Verification items for the finished model (mm, model axes). A direction names the side the tool comes from. Coordinates: 2 decimals unless noted, no trailing zeros. Order: outer loops, then holes, each group sorted by start corner. A loop starts at its lowest first (then second) coordinate and runs counter-clockwise, first axis right, second up. Notation, with made-up numbers: (74, 51) -> (118, 51) arc R33 cw to (118, 88) -> close; hole circle Ø5 at (-12, 54). An arc over 180 degrees is marked (long way). Write item = value, one per line. Start each with the question number.
1. Cross-section at C-C on z = 4.5. Record the cut outline in (x, y), plus the area to 3 significant figures.
2. Cross-section at D-D on x = -6. Record the cut outline in (y, z).
3. Release check for a two-part mould opening along Y. For faces 3 (the cylindrical face through (-19.98, -0.88, 3.54)), 4 (the cylindrical face through (-0.715, -7.375, 3.451)), 5 (the flat face through (-5, 5, 0)) record: +Y half, -Y half, draft (parallel to the pull), parting line (faces both ways), or undercut.
4. Thickness scan on line 1 along Z through (x, y) = (-2.5, 21.5); line 2 along Y through (x, z) = (-5, 2); line 3 along Y through (x, z) = (-6, 1.5). Record the ranges inside material, lowest first. Write a range as from..to.
5. Cross-section at A-A on y = 0. Record the cut outline in (x, z), plus the area to 3 significant figures.
6. Set-up check for faces 1 (the flat face through (-11, -17, 1)), 2 (the cylindrical face through (23.846, -7.509, 6.507)): record each of +Z, -Z, +X, -X, +Y, -Y from which the full face is reachable in a straight line by a thin tool's end or side.
7. Go/stop test with flat-tipped pins: P1, Ø1, axis at x = -1.5, z = 2.5, coming from the +Y side (3 decimals); P2, Ø4, axis at y = 7, z = 3.5, coming from the +X side; P3, Ø1.9, axis at x = 0, y = -6, coming from the +Z side; P4, Ø4, axis at x = -16.5, z = 1.5, coming from the -Y side. Record where each tip stops, or that it passes through.
from build123d import *

# Parameters (mm, degrees)
SKETCH4_R          = 1.55
SKETCH4_R_2        = 2.45
CUT_EXTRUDE1_DEPTH = 37.041642582


with BuildPart() as part:
    # Sketch3 → Revolve2 (revolve)
    with BuildSketch(Plane(origin=(0, 0, 0), x_dir=(1, 0, 0), z_dir=(0, 1, 0)), mode=Mode.PRIVATE) as revolve2_sk:
        Polygon((0, 0), (-25, 0), (-25, -1), (-20, -1), (-20, -6), (-25, -6), (-25, -7), (0, -7), align=None)
    revolve(revolve2_sk.sketch.rotate(Axis((0, 0, 7), (0, 0, -1)), 180), axis=Axis((0, 0, 7), (0, 0, -1)))

    # Sketch4 → Cut-Extrude1 (cut, through all)
    with BuildSketch(Plane(origin=(0, 0, 0), x_dir=(-1, 0, 0), z_dir=(0, 0, -1))):
        with Locations((0, 6)):
            Circle(SKETCH4_R)
        with Locations((6, 0)):
            Circle(SKETCH4_R)
        with Locations((0, -6)):
            Circle(SKETCH4_R)
        with Locations((-6, 0)):
            Circle(SKETCH4_R)
        Circle(SKETCH4_R_2)
    extrude(amount=-CUT_EXTRUDE1_DEPTH, mode=Mode.SUBTRACT)


solid = part.part
Worked out:
q1.outline = circle Ø40 at (0, 0); hole circle Ø3.1 at (-6, 0); hole circle Ø4.9 at (0, 0); hole circle Ø3.1 at (0, -6); hole circle Ø3.1 at (0, 6); hole circle Ø3.1 at (6, 0)
q1.area = 1,210 mm²
q2.outline = (-24.27, 0) -> (-1.55, 0) -> (-1.55, 7) -> (-24.27, 7) -> (-24.27, 6) -> (-19.08, 6) -> (-19.08, 1) -> (-24.27, 1) -> close; (1.55, 0) -> (24.27, 0) -> (24.27, 1) -> (19.08, 1) -> (19.08, 6) -> (24.27, 6) -> (24.27, 7) -> (1.55, 7) -> close
q3.face_3 = parting line
q3.face_4 = undercut
q3.face_5 = draft
q4.line_1 = 0..1, 6..7
q4.line_2 = -19.36..-1.18, 1.18..19.36
q4.line_3 = -19.08..-1.55, 1.55..19.08
q5.outline = (-25, 0) -> (-7.55, 0) -> (-7.55, 7) -> (-25, 7) -> (-25, 6) -> (-20, 6) -> (-20, 1) -> (-25, 1) -> close; (-4.45, 0) -> (-2.45, 0) -> (-2.45, 7) -> (-4.45, 7) -> close; (2.45, 0) -> (4.45, 0) -> (4.45, 7) -> (2.45, 7) -> close; (7.55, 0) -> (25, 0) -> (25, 1) -> (20, 1) -> (20, 6) -> (25, 6) -> (25, 7) -> (7.55, 7) -> close
q5.area = 222 mm²
q6.face_1 = none
q6.face_2 = +Z, -Z
q7.P1 = 19.975
q7.P2 = 19.36
q7.P3 = through
q7.P4 = -20.32
